Here's how the part is built. I have some questions about the finished solid (model axes, mm). Round coordinates to 2 decimals unless told otherwise and drop trailing zeros. Write each loop counter-clockwise with the first axis right and the second up, starting at its lowest first coordinate (ties: lowest second). Pieces come first, ordered by that corner, then holes. Notation, with made-up numbers: (4.5, 25.5) - (54.5, 25.5) arc R24 ccw to (54.5, 56.5) - close; hole circle Ø8 at (89, 82.25). An arc over 180 degrees is marked (long way). Use one line per item in the form item = value. Start each with the question number.
1. Will these pins go through, and if not, where does the flat tip stop? pin 1 (1.5 mm diameter, centred on y = 0, z = 88, fed in from -X); pin 2 (1 mm diameter, centred on y = 1, z = 11.5, fed in from -X); pin 3 (1.5 mm diameter, centred on x = -16.5, y = 0.5, fed in from -Z).
2. If I drill on line 1 along X through (y, z) = (-0.8, 3.5); line 2 along X through (y, z) = (-0.5, 27); line 3 along Z through (x, y) = (7, 0.9), over which ranges is the centre line in solid material (lowest first)?
3. I want a section at A-A, the plane y = -0.85. List the corners of the cut face in (x, z) for me.
```python
from build123d import *

# Parameters (mm, degrees)
F0_R     = 1.27
F2_W     = 246.2176010013
F2_H     = 106.0751006007
F3_DEPTH = 25.4
F4_DEPTH = 51.308
F6_ANGLE = 90
F7_R     = 1.27
F8_ANGLE = 90


with BuildPart() as f1:
    # F0 (on Top) → F1 (revolve)
    with BuildSketch(Plane.XY):
        with Locations((-101.6, 0)):
            Circle(F0_R)
    revolve(axis=Axis((0, 8.5233533755, 0), (0, 1, 0)))

    # F2 (on Front) → F3 (cut)
    with BuildSketch(Plane.XZ):
        with Locations((10.4999132454, -53.0375503004)):
            Rectangle(F2_W, F2_H)
    extrude(amount=-F3_DEPTH, mode=Mode.SUBTRACT)

    # F2 (on Front) → F4 (cut)
    with BuildSketch(Plane.XZ):
        with Locations((10.4999132454, -53.0375503004)):
            Rectangle(F2_W, F2_H)
    extrude(amount=F4_DEPTH, mode=Mode.SUBTRACT)

    # F5 (on face) → F6 (revolve)
    with BuildSketch(Plane(origin=(0, 0, 0), x_dir=(1, 0, 0), z_dir=(0, 0, -1))):
        with BuildLine():
            ThreePointArc((100.33, 0), (101.6, -1.27), (102.87, 0))
            ThreePointArc((102.87, 0), (101.6, 1.27), (100.33, 0))
        make_face()
    revolve(axis=Axis((93.98, -0.709965534, 0), (0, 1, 0)), revolution_arc=F6_ANGLE)

    # F7 (on face) → F8 (revolve)
    with BuildSketch(Plane(origin=(0, 0, 0), x_dir=(1, 0, 0), z_dir=(0, 0, -1))):
        with Locations((-101.6, 0)):
            Circle(F7_R)
    revolve(axis=Axis((-93.98, -1.0185919236, 0), (0, -1, 0)), revolution_arc=F8_ANGLE)


solid = f1.part
```
Model answer:
q1.pin_1 = -54.49
q1.pin_2 = -102.13
q1.pin_3 = 98.86
q2.line_1 = -102.53 to -100.55, 100.55 to 102.53
q2.line_2 = -99.16 to -96.74, 96.74 to 99.16
q2.line_3 = 100.46 to 102.26
q3.outline = (-102.54, 0) arc R8.56 ccw to (-93.98, -8.56) - (-93.98, -6.68) arc R6.68 cw to (-100.66, 0) arc R100.66 cw to (100.66, 0) arc R6.68 cw to (93.98, -6.68) - (93.98, -8.56) arc R8.56 ccw to (102.54, 0) arc R102.54 ccw to start
